Read the model definition and answer for the solid it produces. Units are mm, in the model's axes. A direction names the side the tool comes from. Give positions to 0.01 mm unless a question says otherwise; leave off trailing zeros. Loops run counter-clockwise (first coordinate to the right, second up) from the corner with the lowest first, then second, coordinate; pieces in that order, holes last. Notation, with made-up numbers: (-36, -18) - (10, -18) arc R24 cw to (10, -5) - close; hole circle Ø5 at (-21.75, 85.5). An arc over 180 degrees is marked (long way). Use a Markdown table: item, result. Add a question column.
Item 1: Which of the six approach directions +Z, -Z, +X, -X, +Y, -Y give full straight-line access (tool end or side, diameter ignored) to faces 1 (the face through (18.6, 1.8, -1.1)), 2 (the face through (0.285, 1.873, -4.699)), 3 (the face through (0.301, 1.873, -0.285)), 4 (the face through (9, 2, 0))?
Item 2: A cutting plane is placed at B-B (y = 3.2). Determine the outline of the cut face in (x, z), plus the area to 3 significant figures.
Item 3: A cutting plane is placed at A-A (x = 14.5). Determine the outline of the cut face in (y, z).
Item 4: Each of these flat-tipped pins is pushed along its axis until it touches: P1, Ø1.5, axis at x = 16, y = 1.5, coming from the +Z side; P2, Ø1, axis at x = 9, y = 1, coming from the -Z side; P3, Ø4, axis at x = 3.5, z = -5, coming from the +Y side; P4, Ø0.9, axis at y = 2, z = -2, coming from the -X side. Where does it stop, or does it pass through?
Item 5: Consider probe 1 along Z at (x, y) = (8.75, 2.1); probe 2 along Y at (x, z) = (18.25, -4.5); probe 3 along X at (y, z) = (-0.1, -0.5). Determine where each line is inside the solid, lowest interval first. Write a range as [from, to].
from build123d import *

# Parameters (mm, degrees)
BOSS_EXTRUDE1_DEPTH = 4
FILLET1_R           = 1
FILLET2_R           = 0.5
BOSS_EXTRUDE2_DEPTH = 1
FILLET3_R           = 0.2
FILLET4_R           = 0.2


with BuildPart() as part:
    # Sketch1 → Boss-Extrude1 (new body)
    with BuildSketch(Plane(origin=(0, 0, 0), x_dir=(1, 0, 0), z_dir=(0, 1, 0))):
        Polygon((17.5, 5), (20, 2.5), (17.5, 0), (0, 0), (0, 5), align=None)
    extrude(amount=BOSS_EXTRUDE1_DEPTH)

    # Fillet1
    fillet1_edges = [part.edges().sort_by_distance(p)[0] for p in [
        (0, 2, -5),
        (17.5, 2, -5),
        (20, 2, -2.5),
        (17.5, 2, 0),
        (0, 2, 0),
    ]]
    fillet(fillet1_edges, radius=FILLET1_R)

    # Fillet2
    fillet2_edges = [part.edges().sort_by_distance(p)[0] for p in [
        (9.042893219, 4, -5),
        (18.542893219, 4, -3.957106781),
        (0, 4, -2.5),
        (9.042893219, 4, 0),
        (18.542893219, 4, -1.042893219),
        (19.585786438, 4, -2.5),
        (17.46846987, 4, -0.076120467),
        (0.292893219, 4, -0.292893219),
        (0.292893219, 4, -4.707106781),
        (17.46846987, 4, -4.923879533),
    ]]
    fillet(fillet2_edges, radius=FILLET2_R)

    # Sketch2 → Boss-Extrude2 (add)
    with BuildSketch(Plane.XZ):
        with BuildLine():
            Line((1, -5.9), (17.085786438, -5.9))
            ThreePointArc((17.085786438, -5.9), (17.812884959, -5.755371112), (18.429289322, -5.343502884))
            Line((18.429289322, -5.343502884), (19.929289322, -3.843502884))
            ThreePointArc((19.929289322, -3.843502884), (20.485786438, -2.5), (19.929289322, -1.156497116))
            Line((19.929289322, -1.156497116), (18.429289322, 0.343502884))
            ThreePointArc((18.429289322, 0.343502884), (17.812884959, 0.755371112), (17.085786438, 0.9))
            Line((17.085786438, 0.9), (1, 0.9))
            ThreePointArc((1, 0.9), (-0.343502884, 0.343502884), (-0.9, -1))
            Line((-0.9, -1), (-0.9, -4))
            ThreePointArc((-0.9, -4), (-0.343502884, -5.343502884), (1, -5.9))
        make_face()
    extrude(amount=BOSS_EXTRUDE2_DEPTH)

    # Fillet3
    fillet3_edges = [part.edges().sort_by_distance(p)[0] for p in [
        (9.042893219, 0, -5),
        (0, 0, -2.5),
        (18.542893219, 0, -3.957106781),
        (18.542893219, 0, -1.042893219),
        (9.042893219, 0, 0),
        (19.585786438, 0, -2.5),
        (17.46846987, 0, -0.076120467),
        (0.292893219, 0, -0.292893219),
        (0.292893219, 0, -4.707106781),
        (17.46846987, 0, -4.923879533),
    ]]
    fillet(fillet3_edges, radius=FILLET3_R)

    # Fillet4
    fillet4_edges = [part.edges().sort_by_distance(p)[0] for p in [
        (-0.343502884, 0, -5.343502884),
        (9.042893219, 0, -5.9),
        (17.812884959, 0, -5.755371112),
        (19.179289322, 0, -4.593502884),
        (20.485786438, 0, -2.5),
        (19.179289322, 0, -0.406497116),
        (17.812884959, 0, 0.755371112),
        (9.042893219, 0, 0.9),
        (-0.343502884, 0, 0.343502884),
        (-0.9, 0, -2.5),
    ]]
    fillet(fillet4_edges, radius=FILLET4_R)


solid = part.part
Geometry says:
| question | item | result |
|---|---|---|
| 1 | face 1 | +Z, +X, +Y |
| 1 | face 2 | -Z, -X, +Y |
| 1 | face 3 | +Z, -X, +Y |
| 1 | face 4 | +Z, +X, -X, +Y |
| 2 | outline | (0, -4) arc R1 ccw to (1, -5) - (17.09, -5) arc R1 ccw to (17.79, -4.71) - (19.29, -3.21) arc R1 ccw to (19.29, -1.79) - (17.79, -0.29) arc R1 ccw to (17.09, 0) - (1, 0) arc R1 ccw to (0, -1) - close |
| 2 | area | 93.1 mm² |
| 3 | outline | (-1, -5.9) - (-0.2, -5.9) arc R0.2 ccw to (0, -5.7) - (0, -5.2) arc R0.2 cw to (0.2, -5) - (3.5, -5) arc R0.5 ccw to (4, -4.5) - (4, -0.5) arc R0.5 ccw to (3.5, 0) - (0.2, 0) arc R0.2 cw to (0, 0.2) - (0, 0.7) arc R0.2 ccw to (-0.2, 0.9) - (-1, 0.9) - close |
| 4 | P1 | z = 0 |
| 4 | P2 | z = -5 |
| 4 | P3 | y = 4 |
| 4 | P4 | x = 0 |
| 5 | probe 1 | [-5, 0] |
| 5 | probe 2 | [-1, 0] |
| 5 | probe 3 | [-0.81, 19.23] |
